from build123d import *

# Parameters (mm, degrees)
SKETCH_1_W             = 40
SKETCH_1_H             = 40
EXTRUDE_644_DEPTH      = 8
SKETCH_2_W             = 28.8
SKETCH_2_H             = 29.8
CUT_EXTRUDE_826_DEPTH  = 5.3
SKETCH_3_W             = 28.8
SKETCH_3_H             = 20.86
CUT_EXTRUDE_1017_DEPTH = 29.776552955
SKETCH_4_W             = 12
SKETCH_4_H             = 4.47
CUT_EXTRUDE_1234_DEPTH = 2
SKETCH_5_W             = 28.8
SKETCH_5_H             = 0.5
EXTRUDE_1465_DEPTH     = 4
SKETCH_7_R             = 1.25
CUT_EXTRUDE_1704_DEPTH = 30.393876913
FILLET_1_R             = 2
SKETCH_8_R             = 2.35
CUT_EXTRUDE_2246_DEPTH = 4


with BuildPart() as part:
    # Эскиз1 → Extrude 644 (new body)
    with BuildSketch(Plane(origin=(0, 0, 0), x_dir=(1, 0, 0), z_dir=(0, 1, 0))):
        Rectangle(SKETCH_1_W, SKETCH_1_H)
    extrude(amount=EXTRUDE_644_DEPTH)

    # Эскиз2 → Cut-Extrude 826 (cut)
    with BuildSketch(Plane.XZ):
        Rectangle(SKETCH_2_W, SKETCH_2_H)
    extrude(amount=-CUT_EXTRUDE_826_DEPTH, mode=Mode.SUBTRACT)

    # Эскиз3 → Cut-Extrude 1017 (cut, through all)
    with BuildSketch(Plane.XZ.offset(-5.3)):
        Rectangle(SKETCH_3_W, SKETCH_3_H)
    extrude(amount=-CUT_EXTRUDE_1017_DEPTH, mode=Mode.SUBTRACT)

    # Эскиз4 → Cut-Extrude 1234 (cut)
    with BuildSketch(Plane.XZ.offset(-5.3)):
        with Locations((0, 12.665)):
            Rectangle(SKETCH_4_W, SKETCH_4_H)
        with Locations((0, -12.665)):
            Rectangle(SKETCH_4_W, SKETCH_4_H)
    extrude(amount=-CUT_EXTRUDE_1234_DEPTH, mode=Mode.SUBTRACT)

    # Эскиз5 → Extrude 1465 (add)
    with BuildSketch(Plane(origin=(0, 0, 10.43), x_dir=(-1, 0, 0), z_dir=(0, 0, -1))):
        with Locations((0, 7.75)):
            Rectangle(SKETCH_5_W, SKETCH_5_H)
    extrude(amount=EXTRUDE_1465_DEPTH)

    # Эскиз7 → Cut-Extrude 1704 (cut, through all)
    with BuildSketch(Plane.XZ):
        with Locations(Location((-16.5, 16.5, 0), (0, 0, 270))):
            Circle(SKETCH_7_R)
        with Locations(Location((16.5, 16.5, 0), (0, 0, 270))):
            Circle(SKETCH_7_R)
        with Locations(Location((16.5, -16.5, 0), (0, 0, 270))):
            Circle(SKETCH_7_R)
        with Locations(Location((-16.5, -16.5, 0), (0, 0, 270))):
            Circle(SKETCH_7_R)
    extrude(amount=-CUT_EXTRUDE_1704_DEPTH, mode=Mode.SUBTRACT)

    # Скругление1
    fillet_1_edges = [part.edges().sort_by_distance(p)[0] for p in [
        (20, 4, 20),
        (-20, 4, 20),
        (-20, 4, -20),
        (20, 4, -20),
    ]]
    fillet(fillet_1_edges, radius=FILLET_1_R)

    # Эскиз8 → Cut-Extrude 2246 (cut)
    with BuildSketch(Plane(origin=(0, 8, 0), x_dir=(1, 0, 0), z_dir=(0, 1, 0))):
        with Locations(Location((-16.5, 16.5, 0), (0, 0, 270))):
            Circle(SKETCH_8_R)
        with Locations(Location((-16.5, -16.5, 0), (0, 0, 270))):
            Circle(SKETCH_8_R)
        with Locations(Location((16.5, -16.5, 0), (0, 0, 270))):
            Circle(SKETCH_8_R)
        with Locations(Location((16.5, 16.5, 0), (0, 0, 270))):
            Circle(SKETCH_8_R)
    extrude(amount=-CUT_EXTRUDE_2246_DEPTH, mode=Mode.SUBTRACT)


solid = part.part
Geometry check sheet. Reference: the model listing, model coordinates, mm. A direction names the side the tool comes from. Coordinates: 2 decimals unless noted, no trailing zeros. Loops run counter-clockwise (first coordinate to the right, second up) from the corner with the lowest first, then second, coordinate; pieces in that order, holes last. Notation, with made-up numbers: (22.25, 2) - (40.25, 2) arc R28 ccw to (40.25, 24) - close; hole circle Ø2 at (40.25, 40.5). An arc over 180 degrees is marked (long way). Use one line per item in the form item = value. Start each with the question number.
Item 1: Section check C-C, the plane x = -1. Enter the section's corners in (y, z).
Item 2: Tool access check on faces 4 (the face through (-18, 0, 0)), 5 (the face through (15.07, 6.028, -18.365)), 6 (the face through (6, 6, 13)). Record the directions out of +Z, -Z, +X, -X, +Y, -Y that give a thin tool (end or side, any length) a straight path to the whole face; none if there is none.
Item 3: Section check D-D, the plane y = 0.75. Enter the section's corners in (x, z).
Item 4: Gauge pin test, flat ends, axial feed: pin 1 (3.5 mm diameter, centred on x = -9.5, z = -12.5, fed in from -Y); pin 2 (3.5 mm diameter, centred on x = 1.5, z = -11.5, fed in from -Y). Record the tip position at first contact, or that the pin passes through.
Item 5: Section check B-B, the plane z = 4. Enter the section's corners in (x, y), and give its area (3 significant figures).
Item 6: Thickness scan on probe 1 along X at (y, z) = (6.55, 16.5); probe 2 along X at (y, z) = (2, 0.5); probe 3 along Z at (x, y) = (3.5, 3.75). Record the ranges inside material, lowest first.
Item 7: Mould release check, pull along X, two halves, no side actions. Record for faces 1 (the face through (0, 4, -20)), 2 (the face through (19.4, 4.06, -19.43)), 3 (the face through (-15.26, 1.97, -16.34)): +X half, -X half, draft (parallel to the pull), parting line (faces both ways), or undercut.
Item 8: Section check A-A, the plane x = 16.5. Enter the section's corners in (y, z).
Computed:
q1.outline = (0, -20) - (8, -20) - (8, -10.43) - (7.3, -10.43) - (7.3, -14.9) - (0, -14.9) - close; (0, 14.9) - (7.3, 14.9) - (7.3, 10.43) - (7.5, 10.43) - (7.5, 6.43) - (8, 6.43) - (8, 20) - (0, 20) - close
q2.face_4 = +Z, -Z, +X, -X, -Y
q2.face_5 = +Y
q2.face_6 = -Y
q3.outline = (-20, -18) arc R2 ccw to (-18, -20) - (18, -20) arc R2 ccw to (20, -18) - (20, 18) arc R2 ccw to (18, 20) - (-18, 20) arc R2 ccw to (-20, 18) - close; hole circle Ø2.5 at (-16.5, -16.5); hole circle Ø2.5 at (-16.5, 16.5); hole (-14.4, -14.9) - (14.4, -14.9) - (14.4, 14.9) - (-14.4, 14.9) - close; hole circle Ø2.5 at (16.5, -16.5); hole circle Ø2.5 at (16.5, 16.5)
q4.pin_1 = 5.3
q4.pin_2 = 7.3
q5.outline = (-20, 0) - (-14.4, 0) - (-14.4, 8) - (-20, 8) - close; (14.4, 0) - (20, 0) - (20, 8) - (14.4, 8) - close
q5.area = 89.6 mm2
q6.probe_1 = -20 to -18.85, -14.15 to 14.15, 18.85 to 20
q6.probe_2 = -20 to -14.4, 14.4 to 20
q6.probe_3 = -20 to -14.9, 14.9 to 20
q7.face_1 = draft
q7.face_2 = +X half
q7.face_3 = undercut
q8.outline = (0, -20) - (8, -20) - (8, -18.85) - (4, -18.85) - (4, -17.75) - (0, -17.75) - close; (0, -15.25) - (4, -15.25) - (4, -14.15) - (8, -14.15) - (8, 14.15) - (4, 14.15) - (4, 15.25) - (0, 15.25) - close; (0, 17.75) - (4, 17.75) - (4, 18.85) - (8, 18.85) - (8, 20) - (0, 20) - close
